Design review of the part built by this model. Coordinates are the model's own, in mm. A direction names the side the tool comes from. Give positions to 0.01 mm unless a question says otherwise; leave off trailing zeros. Loops run counter-clockwise (first coordinate to the right, second up) from the corner with the lowest first, then second, coordinate; pieces in that order, holes last. Notation, with made-up numbers: M 61.5,14.5 L 94.5,14.5 A21 ccw 94.5,27.5 Z; hole C 19.5,50.5 d7. An arc over 180 degrees is marked long. Use a Markdown table: item, result. Add a question column.
(1) Add section A-A, the plane y = 50. Give the boundary of the cut face in (x, z).
(2) For faces 1 (the face through (-1, 30, 0)), 2 (the face through (0, 0, 0)), list the 3-axis set-ups (+Z, -Z, +X, -X, +Y, -Y) from which the entire face can be reached by the end or side of a thin tool; tool diameter is ignored.
(3) For probe 1 along X at (y, z) = (41.5, -0.05); probe 2 along Y at (x, z) = (-2.05, 0.1); probe 3 along Z at (x, y) = (-0.15, 55), list the stretches that pass through material, from the lowest coordinate up.
(4) Insertion check: pin 1 Ø2 at (x, z) = (-2.5, 1.5) entering from +Y. The pin has a flat end and moves straight along its axis. Give the tip position at first contact, or say it passes through.
```python
from build123d import *

# Parameters (mm, degrees)
SWEEP1_PROFILE_R    = 1
SKETCH10_R          = 1.9
BOSS_EXTRUDE1_DEPTH = 1.2
CHAMFER1_SIZE       = 1.5
CHAMFER1_SIZE_2     = 0.545955351
FILLET1_R           = 0.5


with BuildPart() as part:
    # Sweep1: sweep along a path in Sketch1
    with BuildLine(Plane.XY) as sweep1_path:
        Line((0, 0), (0, 60))
        ThreePointArc((0, 60), (-0.585786438, 61.414213562), (-2, 62))
        Line((-2, 62), (-3.5, 62))
    # Sweep1 profile (on start of the path) → Sweep1 (sweep)
    with BuildSketch(Plane.ZX):
        Circle(SWEEP1_PROFILE_R)
    sweep(path=sweep1_path.line)

    # Sketch10 → Boss-Extrude1 (add)
    with BuildSketch(Plane.ZY.offset(3.5)):
        with Locations(Location((0, 62, 0), (0, 0, 270))):
            Circle(SKETCH10_R)
    extrude(amount=-BOSS_EXTRUDE1_DEPTH)

    # Chamfer1
    # the kernel refuses this chamfer: 1.5, 0.545955351 mm, written as the material it takes off along each edge
    with BuildSketch(Plane(origin=(-2.3, 62, 0), x_dir=(0, -1, 0), z_dir=(0, 0, -1))) as chamfer1_piece_1_section:
        Polygon((1.9 - CHAMFER1_SIZE, 0), (1.9, CHAMFER1_SIZE_2), (1.9, 0), align=None)
    chamfer1_piece_1 = revolve(axis=Axis((-2.3, 62, 0), (-1, 0, 0)), mode=Mode.PRIVATE)
    chamfer1_piece_1 = chamfer1_piece_1 - Plane(origin=(-2.677798348, 62, 0), x_dir=(0, 0, 1), z_dir=(-1, 0, 0)) * Cylinder(1, 8, mode=Mode.PRIVATE)
    add(chamfer1_piece_1, mode=Mode.SUBTRACT)

    # Fillet1
    fillet1_edges = [part.edges().sort_by_distance(p)[0] for p in [
        (-3.5, 63.9, 0),
        (-2.51838214, 61.292893219, 0.707106781),
    ]]
    fillet(fillet1_edges, radius=FILLET1_R)


solid = part.part
```
Established:
| question | item | result |
|---|---|---|
| 1 | outline | C 0,0 d2 |
| 2 | face 1 | -Y |
| 2 | face 2 | +Z, -Z, +X, -X, -Y |
| 3 | probe 1 | -1 to 1 |
| 3 | probe 2 | 61.01 to 62.99 |
| 3 | probe 3 | -0.99 to 0.99 |
| 4 | pin 1 | y = 63.82 |
